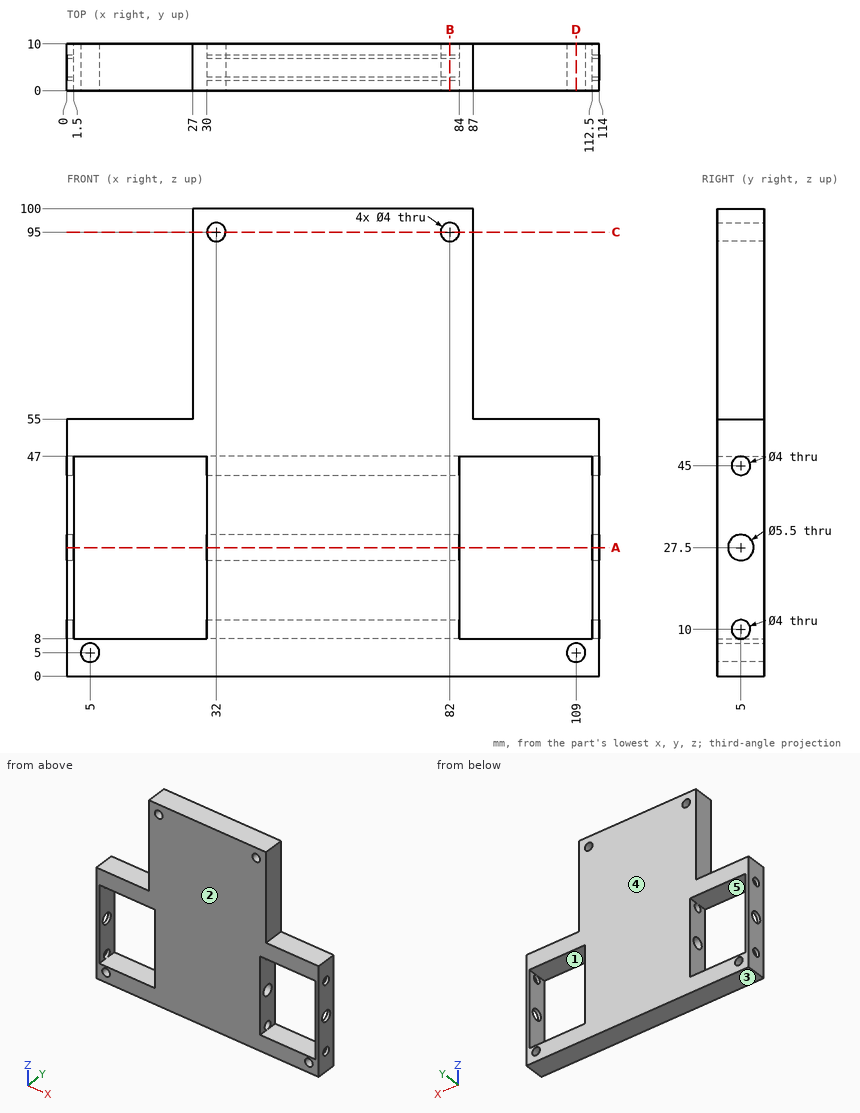
Answer from the drawing. Dimensions are ordinates in mm from the lowest x, y and z of the part. A direction names the side the tool comes from. Coordinates: 2 decimals unless noted, no trailing zeros. Order: outer loops, then holes, each group sorted by start corner. A loop starts at its lowest first (then second) coordinate and runs counter-clockwise, first axis right, second up. Notation, with made-up numbers: (81.25, 74) - (111.25, 74) arc R8 ccw to (111.25, 88) - close; hole circle Ø8 at (47.25, 29.25). An arc over 180 degrees is marked (long way). Answer as a JSON object with one key per item and string values. Group by question number.
Item 1: Section A-A (z = 27.5) is taken. Give the vertices of the cut face in (x, y).
Item 2: A tool of negligible diameter and unlimited length cuts with its end or side. For the marked faces 4 and 5, from which of +Z, -Z, +X, -X, +Y, -Y can it reach the whole face along a straight path? Write none if from no direction.
Item 3: Section D-D (x = 109) is taken. Give the vertices of the cut face in (y, z), plus the area to 3 significant figures.
Item 4: Consider probe 1 along X at (y, z) = (7, 95); probe 2 along X at (y, z) = (1.5, 34); probe 3 along Z at (x, y) = (5, 4.5). Determine where each line is inside the solid, lowest interval first. Write a range as from..to.
Item 5: Flat-ended cylindrical pins translate along their axes: P1, Ø2.5, axis at y = 5, z = 10, coming from the -X side; P2, Ø3, axis at y = 3, z = 86.5, coming from the +X side; P3, Ø3, axis at x = 102, y = 2.5, coming from the +Z side. Find the tip coordinate at first contact, or state that the pin passes through.
Item 6: Section C-C (z = 95) is taken. Give the vertices of the cut face in (x, y), plus the area to 3 significant figures.
Item 7: The mould has two halves that part along Z. Classify the marked faces 1, 2 and 3: +Z half, -Z half, draft (parallel to the pull), parting line (faces both ways), or undercut.
Item 8: Section B-B (x = 82) is taken. Give the vertices of the cut face in (y, z).
Results are:
{
 "1": {"outline": "(0, 0) - (1.5, 0) - (1.5, 2.25) - (0, 2.25) - close; (0, 7.75) - (1.5, 7.75) - (1.5, 10) - (0, 10) - close; (30, 0) - (84, 0) - (84, 2.25) - (30, 2.25) - close; (30, 7.75) - (84, 7.75) - (84, 10) - (30, 10) - close; (112.5, 0) - (114, 0) - (114, 2.25) - (112.5, 2.25) - close; (112.5, 7.75) - (114, 7.75) - (114, 10) - (112.5, 10) - close"},
 "2": {"face 4": "+Z, -Z, +X, -X, +Y", "face 5": "+Y, -Y"},
 "3": {"outline": "(0, 0) - (10, 0) - (10, 3) - (0, 3) - close; (0, 7) - (10, 7) - (10, 8) - (0, 8) - close; (0, 47) - (10, 47) - (10, 55) - (0, 55) - close", "area": "120 mm^2"},
 "4": {"probe 1": "x = 27..30, 34..80, 84..87", "probe 2": "x = 0..1.5, 30..84, 112.5..114", "probe 3": "z = 0..3, 7..8, 47..55"},
 "5": {"P1": "passes through", "P2": "stops at x = 87", "P3": "stops at z = 55"},
 "6": {"outline": "(27, 0) - (30, 0) - (30, 10) - (27, 10) - close; (34, 0) - (80, 0) - (80, 10) - (34, 10) - close; (84, 0) - (87, 0) - (87, 10) - (84, 10) - close", "area": "520 mm^2"},
 "7": {"face 1": "undercut", "face 2": "draft", "face 3": "-Z half"},
 "8": {"outline": "(0, 0) - (10, 0) - (10, 93) - (0, 93) - close; (0, 97) - (10, 97) - (10, 100) - (0, 100) - close; hole circle Ø5.5 at (5, 27.5); hole circle Ø4 at (5, 10); hole circle Ø4 at (5, 45)"}
}
